Geometry: final body of the model. Coordinates: model frame, mm. A direction names the side the tool comes from. Give positions to 0.01 mm unless a question says otherwise; leave off trailing zeros. Write each loop counter-clockwise with the first axis right and the second up, starting at its lowest first coordinate (ties: lowest second). Pieces come first, ordered by that corner, then holes. Notation, with made-up numbers: M 3,-20.75 L 13,-20.75 A22 cw 13,-2.75 Z; hole C 43.25,42.25 d10. An arc over 180 degrees is marked long. Answer as a JSON object with one key per item and string values.
from build123d import *

# Parameters (mm, degrees)
SKETCH_1_W          = 150
SKETCH_1_H          = 110
EXTRUDE_1_DEPTH     = 12
FILLET_1_R          = 12.5
SHELL_1_T           = -5
SKETCH_3_R          = 2.25
CUT_EXTRUDE_1_DEPTH = 94.268429814


with BuildPart() as part:
    # 草图1 → 凸台-拉伸1 (new body)
    with BuildSketch(Plane.XY):
        Rectangle(SKETCH_1_W, SKETCH_1_H)
    extrude(amount=EXTRUDE_1_DEPTH)

    # 圆角1
    fillet_1_edges = [part.edges().sort_by_distance(p)[0] for p in [
        (75, -55, 6),
        (-75, -55, 6),
        (-75, 55, 6),
        (75, 55, 6),
    ]]
    fillet(fillet_1_edges, radius=FILLET_1_R)

    # 抽壳1
    shell_1_openings = [part.faces().sort_by_distance(p)[0] for p in [
        (0, 0, 12),
    ]]
    offset(amount=SHELL_1_T, openings=shell_1_openings, kind=Kind.INTERSECTION)

    # 草图3 → 切除-拉伸1 (cut, through all)
    with BuildSketch(Plane.XY.offset(5)):
        with Locations((-60, 40)):
            Circle(SKETCH_3_R)
        with Locations((60, 40)):
            Circle(SKETCH_3_R)
        with Locations(Location((60, -40, 0), (0, 0, 180))):
            Circle(SKETCH_3_R)
        with Locations(Location((-60, -40, 0), (0, 0, 180))):
            Circle(SKETCH_3_R)
    extrude(amount=-CUT_EXTRUDE_1_DEPTH, mode=Mode.SUBTRACT)


solid = part.part
1) Cut plane A-A on y = -40. Return loops of the section in (x, z).
Geometry check:
{"outline": "M -75,0 L -62.25,0 L -62.25,5 L -70,5 L -70,12 L -75,12 Z; M -57.75,0 L 57.75,0 L 57.75,5 L -57.75,5 Z; M 62.25,0 L 75,0 L 75,12 L 70,12 L 70,5 L 62.25,5 Z"}
2) Cut plane D-D on x = 15.5. Return loops of the section in (y, z), and give its area (3 significant figures).
Geometry check:
{"outline": "M -55,0 L 55,0 L 55,12 L 50,12 L 50,5 L -50,5 L -50,12 L -55,12 Z", "area": "620 mm2"}
3) Cut plane C-C on y = -17. Return loops of the section in (x, z), and give its area (3 significant figures).
Geometry check:
{"outline": "M -75,0 L 75,0 L 75,12 L 70,12 L 70,5 L -70,5 L -70,12 L -75,12 Z", "area": "820 mm2"}
4) Line query: line 1 (Y direction, x = 60, z = 3.3); line 2 (X direction, y = -40, z = 3.25); line 3 (X direction, y = 30.5, z = 7). Output: solid intervals per line, ascending. Write a range as from..to.
Geometry check:
{"line 1": "y = -55..-42.25, -37.75..37.75, 42.25..55", "line 2": "x = -75..-62.25, -57.75..57.75, 62.25..75", "line 3": "x = -75..-70, 70..75"}
5) Pull-direction query (X, two-part tool) for faces 3 (the flat face through (-1, 55, 6)), 4 (the cylindrical face through (59.71, 42.23, 2.54)), 5 (the cylindrical face through (71.241, -51.435, 6.084)), 6 (the flat face through (70, -1, 8)); classes: pulls with the +X half, pulls with the -X half, needs draft (parallel to the pull), parting line crosses it, or undercut.
Geometry check:
{"face 3": "needs draft", "face 4": "undercut", "face 5": "pulls with the +X half", "face 6": "undercut"}
6) Set-up query: faces 1 (the flat face through (-1, 1, 5)), 2 (the cylindrical face through (61.66, -41.52, 2.54)). Return all of +Z, -Z, +X, -X, +Y, -Y with unobstructed straight access to the full face (end or side cutting, diameter ignored); none if empty.
Geometry check:
{"face 1": "+Z", "face 2": "+Z, -Z"}
7) Contact query for a flat-ended pin moving along its axis: P1, Ø6, axis at x = 0, y = -25, coming from the +Z side. Output: stop coordinate, or through.
Geometry check:
{"P1": "stops at z = 5"}
8) Cut plane B-B on x = -60. Return loops of the section in (y, z), and give its area (3 significant figures).
Geometry check:
{"outline": "M -55,0 L -42.25,0 L -42.25,5 L -50,5 L -50,12 L -55,12 Z; M -37.75,0 L 37.75,0 L 37.75,5 L -37.75,5 Z; M 42.25,0 L 55,0 L 55,12 L 50,12 L 50,5 L 42.25,5 Z", "area": "575 mm2"}
